from build123d import *

# Parameters (mm, degrees)
BOSS_EXTRUDE1_DEPTH = 3
SKETCH2_W           = 3
SKETCH2_H           = 30
CUT_EXTRUDE1_DEPTH  = 321.943920335
SKETCH3_W           = 10
SKETCH3_H           = 6
CUT_EXTRUDE2_DEPTH  = 321.943920335
SKETCH4_R           = 1.5
SKETCH4_W           = 5
SKETCH4_H           = 3
CUT_EXTRUDE3_DEPTH  = 321.943920335
SKETCH5_W           = 5
SKETCH5_H           = 6
CUT_EXTRUDE4_DEPTH  = 321.943920335
FILLET1_R           = 2


with BuildPart() as part:
    # Sketch1 → Boss-Extrude1 (new body)
    with BuildSketch(Plane.XY):
        Polygon((0, 0), (8.5, 0), (8.5, -6), (28.5, -6), (28.5, 0), (37, 0), (37, 48), (70, 48), (70, 45), (100, 45), (100, 48), (133, 48), (133, 0), (157.5, 0), (157.5, -6), (187.5, -6), (187.5, 0), (212, 0), (212, 48), (237.5, 48), (237.5, 45), (262.5, 45), (262.5, 48), (288, 48), (288, 0), (291.5, 0), (291.5, -6), (296.5, -6), (296.5, 0), (300, 0), (300, 37.428932188), (297, 37.428932188), (297, 62.428932188), (300, 62.428932188), (300, 99.857864376), (296.464466094, 103.393398282), (294.343145751, 101.272077939), (287.272077939, 108.343145751), (289.393398282, 110.464466094), (285.857864376, 114), (89.521656958, 114), (80, 60), (0, 60), align=None)
    extrude(amount=BOSS_EXTRUDE1_DEPTH)

    # Sketch2 → Cut-Extrude1 (cut, through all)
    with BuildSketch(Plane(origin=(0, 0, 0), x_dir=(-1, 0, 0), z_dir=(0, 0, -1))):
        Polygon((-87.40573319, 102), (-90.360156449, 101.479055467), (-85.150711119, 71.934822877), (-82.19628786, 72.45576741), align=None)
        with Locations((-1.5, 30)):
            Rectangle(SKETCH2_W, SKETCH2_H)
    extrude(amount=-CUT_EXTRUDE1_DEPTH, mode=Mode.SUBTRACT)

    # Sketch3 → Cut-Extrude2 (cut, through all)
    with BuildSketch(Plane(origin=(0, 0, 0), x_dir=(-1, 0, 0), z_dir=(0, 0, -1))):
        with Locations((-28.5, 8)):
            Rectangle(SKETCH3_W, SKETCH3_H)
        with Locations((-8.5, 8)):
            Rectangle(SKETCH3_W, SKETCH3_H)
    extrude(amount=-CUT_EXTRUDE2_DEPTH, mode=Mode.SUBTRACT)

    # Sketch4 → Cut-Extrude3 (cut, through all)
    with BuildSketch(Plane(origin=(0, 0, 0), x_dir=(-1, 0, 0), z_dir=(0, 0, -1))):
        with Locations((-11, 55)):
            Circle(SKETCH4_R)
        with Locations((-22.5, 55.5)):
            Rectangle(SKETCH4_W, SKETCH4_H)
    extrude(amount=-CUT_EXTRUDE3_DEPTH, mode=Mode.SUBTRACT)

    # Sketch5 → Cut-Extrude4 (cut, through all)
    with BuildSketch(Plane(origin=(0, 0, 0), x_dir=(-1, 0, 0), z_dir=(0, 0, -1))):
        with Locations((-275.357864376, 107)):
            Rectangle(SKETCH5_W, SKETCH5_H)
        with Locations((-265.357864376, 107)):
            Rectangle(SKETCH5_W, SKETCH5_H)
        with Locations((-110.357864376, 107)):
            Rectangle(SKETCH5_W, SKETCH5_H)
        with Locations((-100.357864376, 107)):
            Rectangle(SKETCH5_W, SKETCH5_H)
    extrude(amount=-CUT_EXTRUDE4_DEPTH, mode=Mode.SUBTRACT)

    # Fillet1
    fillet1_edges = [part.edges().sort_by_distance(p)[0] for p in [
        (0, 60, 1.5),
        (89.521656958, 114, 1.5),
        (285.857864376, 114, 1.5),
        (300, 99.857864376, 1.5),
    ]]
    fillet(fillet1_edges, radius=FILLET1_R)


solid = part.part
Geometry check sheet. Reference: the model listing, model coordinates, mm. Give positions to 0.01 mm unless a question says otherwise; leave off trailing zeros. Loops run counter-clockwise (first coordinate to the right, second up) from the corner with the lowest first, then second, coordinate; pieces in that order, holes last. Notation, with made-up numbers: (39.5, 24.25) -> (54.5, 24.25) arc R24 cw to (54.5, 36.25) -> close; hole circle Ø1 at (9, 46). An arc over 180 degrees is marked (long way). Answer in a Markdown table with one row per item. Add a question column.
1) Cross-section at C-C on y = 89.5. Record the boundary of the cut face in (x, z).
2) Cross-section at A-A on z = 2. State how many separate pieces and enclosed holes the cut face has, and give its area (3 significant figures).
3) Gauge pin test, flat ends, axial feed: P1, Ø0.9, axis at x = 141.5, z = 1.5, coming from the -Y side; P2, Ø1.5, axis at x = 275, z = 1, coming from the -Y side; P3, Ø1.5, axis at y = 107.5, z = 1, coming from the +X side. Record the tip position at first contact, or that the pin passes through.
4) Draft check along X on faces 1 (the face through (290.857, 104.758, 1.479)), 2 (the face through (181, 68, 0)). Enter one of: pulls with the +X half, pulls with the -X half, needs draft (parallel to the pull), parting line crosses it, or undercut.
5) Cross-section at B-B on x = 203. Record the boundary of the cut face in (y, z), and give its area (3 significant figures).
6) Material ranges on probe 1 along Y at (x, z) = (11, 2.05); probe 2 along X at (y, z) = (27, 2.8); probe 3 along X at (y, z) = (43, 2.65), recorded low to high. Write a range as from..to.
Outcome:
| question | item | result |
|---|---|---|
| 1 | outline | (88.25, 0) -> (300, 0) -> (300, 3) -> (88.25, 3) -> close |
| 2 | separate pieces | 1 |
| 2 | enclosed holes | 8 |
| 2 | area | 21,200 mm^2 |
| 3 | P1 | stops at y = 0 |
| 3 | P2 | stops at y = 48 |
| 3 | P3 | stops at x = 288.87 |
| 4 | face 1 | undercut |
| 4 | face 2 | needs draft |
| 5 | outline | (0, 0) -> (114, 0) -> (114, 3) -> (0, 3) -> close |
| 5 | area | 342 mm^2 |
| 6 | probe 1 | y = -6..5, 11..53.5, 56.5..60 |
| 6 | probe 2 | x = 3..37, 133..212, 288..300 |
| 6 | probe 3 | x = 3..37, 133..212, 288..297 |
